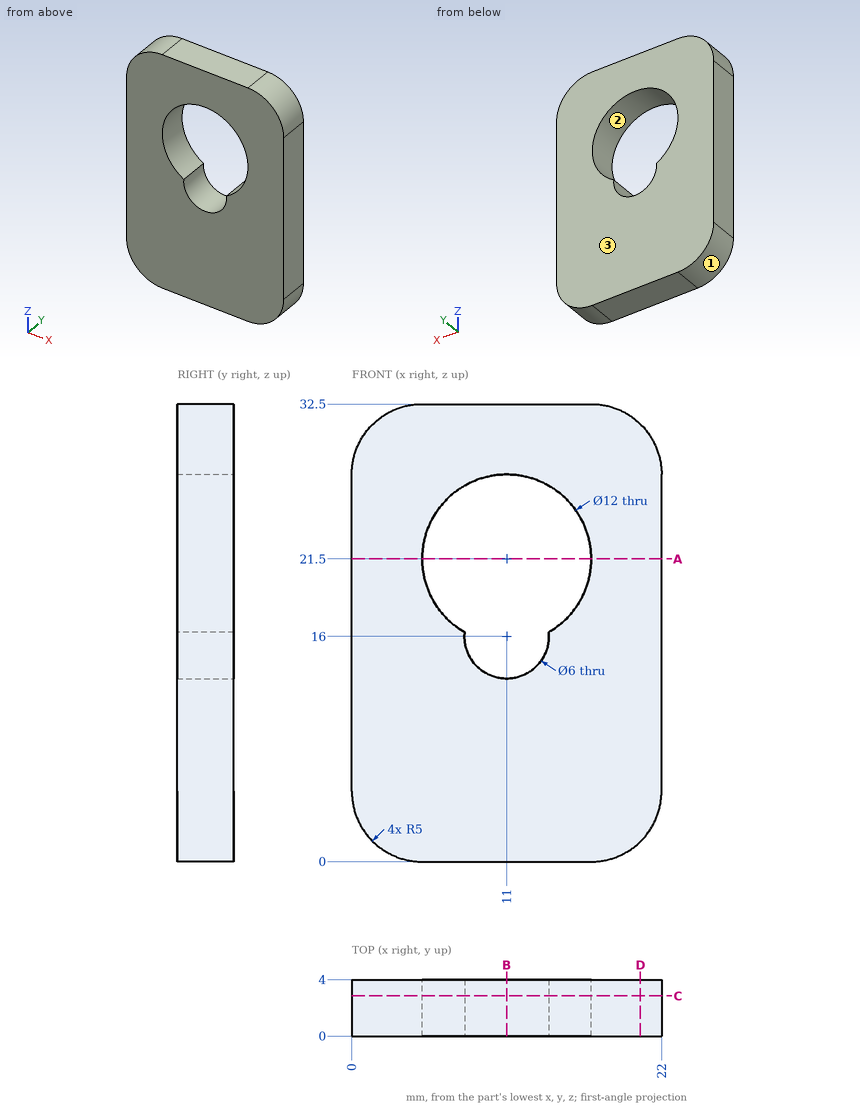
Geometry check sheet. Reference: drawing and pictorial views, mm from the part's lowest x, y, z. Round coordinates to 2 decimals unless told otherwise and drop trailing zeros. Loops run counter-clockwise (first coordinate to the right, second up) from the corner with the lowest first, then second, coordinate; pieces in that order, holes last. Notation, with made-up numbers: (-10, -29) -> (45, -29) arc R26 cw to (45, -15) -> close; hole circle Ø9 at (58, -28). An arc over 180 degrees is marked (long way). Answer as a JSON object with one key per item and string values. Group by question number.
Item 1: Release check for a two-part mould opening along X. For the marked faces 1, 2 and 3 record: pulls with the +X half, pulls with the -X half, needs draft (parallel to the pull), parting line crosses it, or undercut.
Item 2: Cross-section at C-C, the plane y = 2.85. Record the cut outline in (x, z).
Item 3: Depth check by flat-ended pin: pin 1 Ø5.5 at (x, z) = (11, 16) entering from -Y. Enter the tip coordinate at first touch or a pass-through.
Item 4: Cross-section at D-D, the plane x = 20.5. Record the cut outline in (y, z).
Item 5: Cross-section at B-B, the plane x = 11. Record the cut outline in (y, z).
Item 6: Thickness scan on line 1 along Z through (x, y) = (11, 2.7); line 2 along X through (y, z) = (2, 16); line 3 along X through (y, z) = (2.35, 21.5). Record the ranges inside material, lowest first.
Item 7: Cross-section at A-A, the plane z = 21.5. Record the cut outline in (x, y).
Determined:
{
 "1": {"face 1": "pulls with the -X half", "face 2": "undercut", "face 3": "needs draft"},
 "2": {"outline": "(0, 5) arc R5 ccw to (5, 0) -> (17, 0) arc R5 ccw to (22, 5) -> (22, 27.5) arc R5 ccw to (17, 32.5) -> (5, 32.5) arc R5 ccw to (0, 27.5) -> close; hole (8.01, 16.3) arc R3 ccw (long way) to (13.99, 16.3) arc R6 ccw (long way) to start"},
 "3": {"pin 1": "passes through"},
 "4": {"outline": "(0, 1.43) -> (4, 1.43) -> (4, 31.07) -> (0, 31.07) -> close"},
 "5": {"outline": "(0, 0) -> (4, 0) -> (4, 13) -> (0, 13) -> close; (0, 27.5) -> (4, 27.5) -> (4, 32.5) -> (0, 32.5) -> close"},
 "6": {"line 1": "z = 0 to 13, 27.5 to 32.5", "line 2": "x = 0 to 8, 14 to 22", "line 3": "x = 0 to 5, 17 to 22"},
 "7": {"outline": "(0, 0) -> (5, 0) -> (5, 4) -> (0, 4) -> close; (17, 0) -> (22, 0) -> (22, 4) -> (17, 4) -> close"}
}
